```python
from build123d import *

# Parameters (mm, degrees)
BOSS_EXTRUDE1_DEPTH = 10


with BuildPart() as part:
    # Sketch1 → Boss-Extrude1 (new body)
    with BuildSketch(Plane.XY):
        with BuildLine():
            Line((17.5, 78.07327943), (24.5, 78.07327943))
            Line((24.5, 78.07327943), (24.5, 73.287247591))
            Line((24.5, 73.287247591), (-24.5, 73.287247591))
            Line((-24.5, 73.287247591), (-24.5, 78.07327943))
            Line((-24.5, 78.07327943), (-17.5, 78.07327943))
            ThreePointArc((-17.5, 78.07327943), (-15.378679656, 78.951959087), (-14.5, 81.07327943))
            Line((-14.5, 81.07327943), (-14.5, 84.887247591))
            ThreePointArc((-14.5, 84.887247591), (0, 99.387247591), (14.5, 84.887247591))
            Line((14.5, 84.887247591), (14.5, 81.07327943))
            ThreePointArc((14.5, 81.07327943), (15.378679656, 78.951959087), (17.5, 78.07327943))
        make_face()
        with BuildLine():
            ThreePointArc((11.5, 84.887247591), (0, 96.387247591), (-11.5, 84.887247591))
            ThreePointArc((-11.5, 84.887247591), (0, 73.387247591), (11.5, 84.887247591))
        make_face(mode=Mode.SUBTRACT)
    extrude(amount=BOSS_EXTRUDE1_DEPTH)


solid = part.part
```
Source: CAD feature listing. Evaluate the final solid. Frame: model axes, mm. A direction names the side the tool comes from. Coordinates: 2 decimals unless noted, no trailing zeros. Write each loop counter-clockwise with the first axis right and the second up, starting at its lowest first coordinate (ties: lowest second). Pieces come first, ordered by that corner, then holes. Notation, with made-up numbers: M 46.25,51 L 92.25,51 A30 ccw 92.25,73 Z; hole C 25,1.25 d5. An arc over 180 degrees is marked long. Answer as a JSON object with one key per item and string values.
1. Cut plane B-B on z = 1. Output: boundary loops of the cut face in (x, y).
Evaluation:
{"outline": "M -24.5,73.29 L 24.5,73.29 L 24.5,78.07 L 17.5,78.07 A3 cw 14.5,81.07 L 14.5,84.89 A14.5 ccw -14.5,84.89 L -14.5,81.07 A3 cw -17.5,78.07 L -24.5,78.07 Z; hole C 0,84.89 d23"}
2. Cut plane A-A on x = 0. Output: boundary loops of the cut face in (y, z), plus the area to 3 significant figures.
Evaluation:
{"outline": "M 73.29,0 L 73.39,0 L 73.39,10 L 73.29,10 Z; M 96.39,0 L 99.39,0 L 99.39,10 L 96.39,10 Z", "area": "31.0 mm^2"}
3. Access query for faces 4 (the flat face through (-21, 78.073, 5)), 5 (the flat face through (21, 78.073, 5)), 6 (the flat face through (24.5, 76, 5)). Directions: +Z, -Z, +X, -X, +Y, -Y. A direction counts if a zero-diameter tool reaches every point of the face in a straight line with its end or side. Return the directions, or none.
Evaluation:
{"face 4": "+Z, -Z, -X, +Y", "face 5": "+Z, -Z, +X, +Y", "face 6": "+Z, -Z, +X, +Y, -Y"}
4. Contact query for flat-ended pins moving along their axis: P1, Ø5, axis at y = 94, z = 4.5, coming from the -X side; P2, Ø1.9, axis at y = 83.5, z = 2.5, coming from the +X side; P3, Ø3, axis at y = 82.5, z = 7.5, coming from the -X side; P4, Ø2, axis at x = -14.5, y = 94.5, coming from the +Z side. Output: stop coordinate, or through.
Evaluation:
{"P1": "x = -12.9", "P2": "x = 14.5", "P3": "x = -14.5", "P4": "through"}
5. Ray query, L1, parallel to X at y = 75.5, z = 4.5; L2, parallel to Y at x = 7.5, z = 3; L3, parallel to Y at x = -3, z = 7.25. Return the intervals inside material, ascending.
Evaluation:
{"L1": "-24.5 to -6.64, 6.64 to 24.5", "L2": "73.29 to 76.17, 93.61 to 97.3", "L3": "73.29 to 73.79, 95.99 to 99.07"}
6. Draft query along X for faces 1 (the cylindrical face through (15.355, 78.975, 4.93)), 2 (the flat face through (-24.5, 76, 5)), 3 (the cylindrical face through (1.497, 73.485, 4.93)). Return one class per face: released by +X, released by -X, zero draft, split by the parting line, or undercut.
Evaluation:
{"face 1": "released by +X", "face 2": "released by -X", "face 3": "undercut"}
7. Cut plane C-C on y = 85.75. Output: boundary loops of the cut face in (x, z), plus the area to 3 significant figures.
Evaluation:
{"outline": "M -14.47,0 L -11.47,0 L -11.47,10 L -14.47,10 Z; M 11.47,0 L 14.47,0 L 14.47,10 L 11.47,10 Z", "area": "60.1 mm^2"}
